Work out the finished part from the listing and answer in its coordinate system (mm). A direction names the side the tool comes from. Give positions to 0.01 mm unless a question says otherwise; leave off trailing zeros. Loops run counter-clockwise (first coordinate to the right, second up) from the corner with the lowest first, then second, coordinate; pieces in that order, holes last. Notation, with made-up numbers: M 2,89 L 46,89 A29 ccw 46,114 Z; hole C 58.5,64.25 d5. An arc over 180 degrees is marked long. Answer in a Markdown table with one row per item. Add a question column.
from build123d import *

# Parameters (mm, degrees)
F0_W     = 152.4
F0_H     = 304.8
F1_DEPTH = 50.8
F2_W     = 137.16
F2_H     = 63.5
F2_H_2   = 203.2
F3_DEPTH = 82.55
F4_W     = 12.7
F4_H     = 12.7
F5_DEPTH = 7.62


with BuildPart() as f1:
    # F0 (on Front) → F1 (new body, symmetric)
    with BuildSketch(Plane.XZ):
        Rectangle(F0_W, F0_H)
    extrude(amount=F1_DEPTH, both=True)

    # F2 (on face) → F3 (cut)
    with BuildSketch(Plane.XZ.offset(50.8)):
        with Locations((1.597112, 115.759528)):
            Rectangle(F2_W, F2_H)
        with Locations((1.597112, -37.619612)):
            Rectangle(F2_W, F2_H_2)
    extrude(amount=-F3_DEPTH, mode=Mode.SUBTRACT)

    # F4 (on face) → F5 (join)
    with BuildSketch(Plane(origin=(0, 0, -152.4), x_dir=(1, 0, 0), z_dir=(0, 0, -1))):
        with Locations((-69.85, 44.45)):
            Rectangle(F4_W, F4_H)
        with Locations((69.85, 44.45)):
            Rectangle(F4_W, F4_H)
        with Locations((-69.85, -44.45)):
            Rectangle(F4_W, F4_H)
        with Locations((69.85, -44.45)):
            Rectangle(F4_W, F4_H)
    extrude(amount=F5_DEPTH)


solid = f1.part
(1) Which of the six approach directions +Z, -Z, +X, -X, +Y, -Y give full straight-line access (tool end or side, diameter ignored) to faces 4 (the face through (-63.5, -44, -156)), 5 (the face through (-70, -38.1, -156)), 6 (the face through (70, -45, -160.02)), 7 (the face through (1, -10, 63.98))?
(2) Section C-C, the plane z = -87 is taken. Determine the outline of the cut face in (x, y).
(3) Section B-B, the plane y = 24 is taken. Determine the outline of the cut face in (x, z).
(4) Section A-A, the plane x = 9.5 is taken. Determine the outline of the cut face in (y, z).
(5) The mould has two halves that part along X. Classify faces 1 (the face through (70.177, -10, 115)), 2 (the face through (-70, 44, -160.02)), 3 (the face through (76.2, -1, -6)): pulls with the +X half, pulls with the -X half, needs draft (parallel to the pull), parting line crosses it, or undercut.
(6) Each of these flat-tipped pins is pushed along its axis until it touches: P1, Ø12, axis at x = -55.5, z = -92.5, coming from the -Y side; P2, Ø25, axis at x = 24, y = 10.5, coming from the -Z side. Where does it stop, or does it pass through?
(7) Consider line 1 along Z through (x, y) = (-26.5, -12); line 2 along X through (y, z) = (-36, 53); line 3 along Z through (x, y) = (8, 37). Determine where each line is inside the solid, lowest interval first. Write a range as from..to.
Numbers:
| question | item | result |
|---|---|---|
| 1 | face 4 | -Z, +Y, -Y |
| 1 | face 5 | -Z, +X, -X |
| 1 | face 6 | -Z, +X, -X, +Y, -Y |
| 1 | face 7 | -Y |
| 2 | outline | M -76.2,-50.8 L -66.98,-50.8 L -66.98,31.75 L 70.18,31.75 L 70.18,-50.8 L 76.2,-50.8 L 76.2,50.8 L -76.2,50.8 Z |
| 3 | outline | M -76.2,-152.4 L 76.2,-152.4 L 76.2,152.4 L -76.2,152.4 Z; hole M -66.98,-139.22 L 70.18,-139.22 L 70.18,63.98 L -66.98,63.98 Z; hole M -66.98,84.01 L 70.18,84.01 L 70.18,147.51 L -66.98,147.51 Z |
| 4 | outline | M -50.8,-152.4 L 50.8,-152.4 L 50.8,152.4 L -50.8,152.4 L -50.8,147.51 L 31.75,147.51 L 31.75,84.01 L -50.8,84.01 L -50.8,63.98 L 31.75,63.98 L 31.75,-139.22 L -50.8,-139.22 Z |
| 5 | face 1 | undercut |
| 5 | face 2 | needs draft |
| 5 | face 3 | pulls with the +X half |
| 6 | P1 | stops at y = 31.75 |
| 6 | P2 | stops at z = -152.4 |
| 7 | line 1 | z = -152.4..-139.22, 63.98..84.01, 147.51..152.4 |
| 7 | line 2 | x = -76.2..-66.98, 70.18..76.2 |
| 7 | line 3 | z = -152.4..152.4 |
